For this review, take the finished solid that the model builds, in its own axes (mm). Face numbers are marked on the shaded views. Round coordinates to 2 decimals unless told otherwise and drop trailing zeros. Write item = value, one per line. Start each with the question number.
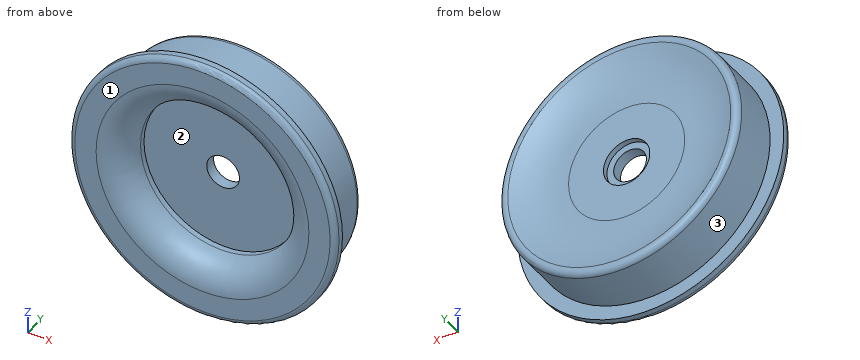
```python
from build123d import *

# Parameters (mm, degrees)
FILLET1_R = 10


with BuildPart() as part:
    # Sketch1 → Revolve1 (revolve)
    with BuildSketch(Plane.XY):
        with BuildLine():
            Line((29, 0), (46.8, 0))
            ThreePointArc((46.8, 0), (48.214213562, 0.585786438), (48.8, 2))
            Line((48.8, 2), (48.8, 4))
            Line((48.8, 4), (43.8, 4))
            Line((43.8, 4), (43.8, 20.522937023))
            ThreePointArc((43.8, 20.522937023), (42.835126597, 22.234226867), (40.871487071, 22.294338655))
            ThreePointArc((40.871487071, 22.294338655), (31.373886886, 18.833953417), (21.3, 18))
            Line((21.3, 18), (8.5, 18))
            Line((8.5, 18), (8.5, 16))
            Line((8.5, 16), (6, 16))
            Line((6, 16), (6, 12))
            Line((6, 12), (29, 12))
            Line((29, 12), (29, 0))
        make_face()
    revolve(axis=Axis((0, 55, 0), (0, -1, 0)))

    # Fillet1
    fillet1_edges = [part.edges().sort_by_distance(p)[0] for p in [
        (-29, 0, 0),
    ]]
    fillet(fillet1_edges, radius=FILLET1_R)


solid = part.part
```
(1) Wall thickness on L1, parallel to Z at x = 0, y = 13.25; L2, parallel to Z at x = 0, y = 11.55; L3, parallel to Y at x = -5.5, z = -12: over which ranges is each line inside the solid? List them lowest first.
(2) Draft analysis for pull direction X (two halves, no side actions). For the marked faces 1, 2 and 3, state which applies: +X half, -X half, draft (parallel to the pull), parting line (faces both ways), or undercut.
(3) For pin 1 Ø1 at (y, z) = (19.5, 28) entering from -X; pin 2 Ø7 at (x, z) = (0, 0) entering from +Y; pin 3 Ø12 at (x, z) = (1.5, -32) entering from +Y; pin 4 Ø5 at (y, z) = (3, -37.5) entering from +X, all flat-tipped, find the tip position at first contact; note any pin that passes through.
Answer sheet:
q1.L1 = -43.8 to -6, 6 to 43.8
q1.L2 = -43.8 to -29, 29 to 43.8
q1.L3 = 12 to 18
q2.face_1 = draft
q2.face_2 = undercut
q2.face_3 = parting line
q3.pin_1 = -34.09
q3.pin_2 = through
q3.pin_3 = 20.95
q3.pin_4 = 34.01
